Geometry: see drawing. Coordinates: mm, zero at the bounding-box minimum. A direction names the side the tool comes from. Round coordinates to 2 decimals unless told otherwise and drop trailing zeros. Loops run counter-clockwise (first coordinate to the right, second up) from the corner with the lowest first, then second, coordinate; pieces in that order, holes last. Notation, with made-up numbers: (68, -34.75) - (99, -34.75) arc R21 cw to (99, -12.75) - close; hole circle Ø1 at (63.25, -8). An arc over 180 degrees is marked (long way). Return JSON: item names as keys, results as strings. Group by question number.
1. First-contact query: pin 1 Ø2.5 at (y, z) = (9.5, 1) entering from -X; pin 2 Ø4 at (x, y) = (22.5, 13) entering from -Z. Flat tips, straight axial feed; report the tip coordinate or a pass-through.
2. Section B-B on x = 56. Return loops of the section in (y, z), and give its area (3 significant figures).
3. Section D-D on y = 13.5. Return loops of the section in (x, z).
4. Set-up query: the marked faces 4 and 5. Return all of +Z, -Z, +X, -X, +Y, -Y with unobstructed straight access to the full face (end or side cutting, diameter ignored); none if empty.
5. Section C-C on y = 5.25. Return loops of the section in (x, z).
6. Material intervals for probe 1 along Y at (x, z) = (56, 5); probe 2 along X at (y, z) = (7.75, 2); probe 3 along X at (y, z) = (7.25, 5.25), sorted ascending.
7. Draft query along X for the marked faces 1, 2 and 3. Return one class per face: +X half, -X half, draft (parallel to the pull), parting line (faces both ways), or undercut.
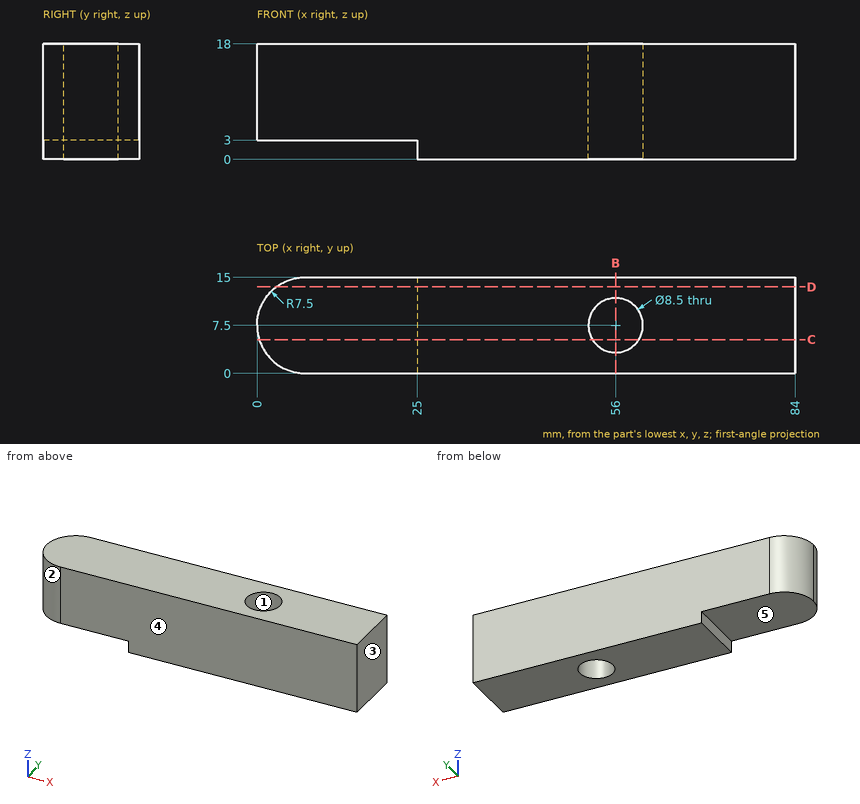
Taken from the geometry:
{
 "1": {"pin 1": "x = 25", "pin 2": "z = 3"},
 "2": {"outline": "(0, 0) - (3.25, 0) - (3.25, 18) - (0, 18) - close; (11.75, 0) - (15, 0) - (15, 18) - (11.75, 18) - close", "area": "117 mm2"},
 "3": {"outline": "(3, 3) - (25, 3) - (25, 0) - (84, 0) - (84, 18) - (3, 18) - close"},
 "4": {"face 4": "+Z, -Z, +X, -X, -Y", "face 5": "-Z, -X, +Y, -Y"},
 "5": {"outline": "(0.35, 3) - (25, 3) - (25, 0) - (52.39, 0) - (52.39, 18) - (0.35, 18) - close; (59.61, 0) - (84, 0) - (84, 18) - (59.61, 18) - close"},
 "6": {"probe 1": "0 to 3.25, 11.75 to 15", "probe 2": "25 to 51.76, 60.24 to 84", "probe 3": "0 to 51.76, 60.24 to 84"},
 "7": {"face 1": "undercut", "face 2": "-X half", "face 3": "+X half"}
}
